Geometry: final body of the model. Coordinates: model frame, mm. A direction names the side the tool comes from. Coordinates: 2 decimals unless noted, no trailing zeros. Write each loop counter-clockwise with the first axis right and the second up, starting at its lowest first coordinate (ties: lowest second). Pieces come first, ordered by that corner, then holes. Notation, with made-up numbers: (36.5, -30) -> (92.5, -30) arc R13 cw to (92.5, -5) -> close; hole circle Ø11 at (38, 88). An arc over 180 degrees is marked (long way). One line per item, written item: value.
```python
from build123d import *

# Parameters (mm, degrees)
SKETCH1_W           = 50.8
SKETCH1_H           = 95.972651844
SKETCH1_R           = 3.175
SKETCH1_R_2         = 3.81
BOSS_EXTRUDE1_DEPTH = 6.35
SKETCH1_3_W         = 6.35
SKETCH1_3_H         = 95.972651844
BOSS_EXTRUDE2_DEPTH = 57.15
FILLET1_R           = 6.35
SKETCH2_R           = 6.096
SKETCH2_R_2         = 2.54
SKETCH2_R_3         = 3.048
CUT_EXTRUDE1_DEPTH  = 6.35
CUT_EXTRUDE2_REACH  = 99.995
SKETCH2_4_R         = 2.54
SKETCH3_W           = 31.75
SKETCH3_H           = 6.35
BOSS_EXTRUDE4_DEPTH = 30.48


with BuildPart() as part:
    # Sketch1 → Boss-Extrude1 (new body)
    with BuildSketch(Plane(origin=(0, 0, 0), x_dir=(1, 0, 0), z_dir=(0, 1, 0))):
        with Locations((0, -0.019674078)):
            Rectangle(SKETCH1_W, SKETCH1_H)
        with Locations(Location((-19.05, -41.656, 0), (0, 0, 270))):
            Circle(SKETCH1_R, mode=Mode.SUBTRACT)
        with Locations(Location((19.05, -41.656, 0), (0, 0, 270))):
            Circle(SKETCH1_R, mode=Mode.SUBTRACT)
        with Locations(Location((-19.05, 41.616651844, 0), (0, 0, 270))):
            Circle(SKETCH1_R, mode=Mode.SUBTRACT)
        with Locations(Location((0, 0, 0), (0, 0, 270))):
            Circle(SKETCH1_R_2, mode=Mode.SUBTRACT)
        with Locations(Location((19.05, 41.616651844, 0), (0, 0, 270))):
            Circle(SKETCH1_R, mode=Mode.SUBTRACT)
    extrude(amount=BOSS_EXTRUDE1_DEPTH)

    # Sketch1<3> → Boss-Extrude2 (add)
    with BuildSketch(Plane(origin=(0, 0, 0), x_dir=(1, 0, 0), z_dir=(0, 1, 0))):
        with Locations((-28.575, -0.019674078)):
            Rectangle(SKETCH1_3_W, SKETCH1_3_H)
        with Locations((28.575, -0.019674078)):
            Rectangle(SKETCH1_3_W, SKETCH1_3_H)
    extrude(amount=BOSS_EXTRUDE2_DEPTH)

    # Fillet1
    # the kernel refuses this fillet: 6.35 mm, written as the material it adds along each edge
    with BuildSketch(Plane(origin=(25.4, 6.35, 48.006), x_dir=(0, 1, 0), z_dir=(0, 0, -1))) as fillet1_piece_1_section:
        with BuildLine():
            CenterArc((FILLET1_R, -FILLET1_R), FILLET1_R, 90, 90)
            Line((0, -FILLET1_R), (0, 0))
            Line((0, 0), (FILLET1_R, 0))
        make_face()
    fillet1_piece_1 = extrude(amount=95.972651844, mode=Mode.PRIVATE)
    fillet1_piece_1 = fillet1_piece_1 - Plane(origin=(19.05, 7.801972373, 41.656), x_dir=(0, 0, 1), z_dir=(0, -1, 0)) * Cylinder(3.175, 218, mode=Mode.PRIVATE)
    fillet1_piece_1 = fillet1_piece_1 - Plane(origin=(19.05, 7.801972373, -41.616651844), x_dir=(0, 0, 1), z_dir=(0, -1, 0)) * Cylinder(3.175, 218, mode=Mode.PRIVATE)
    add(fillet1_piece_1)
    with BuildSketch(Plane(origin=(-25.4, 6.35, -47.966651844), x_dir=(1, 0, 0), z_dir=(0, 0, 1))) as fillet1_piece_2_section:
        with BuildLine():
            CenterArc((FILLET1_R, FILLET1_R), FILLET1_R, 180, 90)
            Line((0, FILLET1_R), (0, 0))
            Line((0, 0), (FILLET1_R, 0))
        make_face()
    fillet1_piece_2 = extrude(amount=95.972651844, mode=Mode.PRIVATE)
    fillet1_piece_2 = fillet1_piece_2 - Plane(origin=(-19.05, 7.801971704, 41.656), x_dir=(0, 0, 1), z_dir=(0, -1, 0)) * Cylinder(3.175, 218, mode=Mode.PRIVATE)
    fillet1_piece_2 = fillet1_piece_2 - Plane(origin=(-19.05, 7.801971704, -41.616651844), x_dir=(0, 0, 1), z_dir=(0, -1, 0)) * Cylinder(3.175, 218, mode=Mode.PRIVATE)
    add(fillet1_piece_2)
    # the kernel refuses this fillet: 6.35 mm, written as the material it takes off along each edge
    with BuildSketch(Plane(origin=(-31.75, 0, -63.841651844), x_dir=(1, 0, 0), z_dir=(0, 0, 1)), Plane(origin=(31.75, 0, 63.881), x_dir=(-1, 0, 0), z_dir=(0, 0, -1))) as fillet1_2_piece_1:
        with BuildLine():
            CenterArc((FILLET1_R, FILLET1_R), FILLET1_R, 180, 90)
            Line((0, FILLET1_R), (0, 0))
            Line((0, 0), (FILLET1_R, 0))
        make_face()
    extrude(amount=127.722651844, mode=Mode.SUBTRACT)

    # Sketch2 → Cut-Extrude1 (cut)
    # profile 1 of 6: a face of its own
    with BuildSketch(Plane(origin=(31.75, 0, 0), x_dir=(0, 0, -1), z_dir=(1, 0, 0))):
        with Locations((-22.606, 31.75)):
            Circle(SKETCH2_R)
        with Locations((-22.606, 31.75)):
            Circle(SKETCH2_R_2, mode=Mode.SUBTRACT)
    # profile 2 of 6: a face of its own
    with BuildSketch(Plane(origin=(31.75, 0, 0), x_dir=(0, 0, -1), z_dir=(1, 0, 0))):
        with Locations((-22.606, 31.75)):
            Circle(SKETCH2_R_2)
    # profile 3 of 6: a face of its own
    with BuildSketch(Plane(origin=(31.75, 0, 0), x_dir=(0, 0, -1), z_dir=(1, 0, 0))):
        with Locations((-22.606, 31.75)):
            Circle(SKETCH2_R)
    # profile 4 of 6: a face of its own
    with BuildSketch(Plane(origin=(31.75, 0, 0), x_dir=(0, 0, -1), z_dir=(1, 0, 0))):
        with Locations((-16.256, 31.75)):
            Circle(SKETCH2_R_3)
    # profile 5 of 6: a face of its own
    with BuildSketch(Plane(origin=(31.75, 0, 0), x_dir=(0, 0, -1), z_dir=(1, 0, 0))):
        with Locations((-22.606, 31.75)):
            Circle(SKETCH2_R)
    # profile 6 of 6: a face of its own
    with BuildSketch(Plane(origin=(31.75, 0, 0), x_dir=(0, 0, -1), z_dir=(1, 0, 0))):
        with Locations((-16.256, 31.75)):
            Circle(SKETCH2_R_3)
    extrude(amount=-CUT_EXTRUDE1_DEPTH, mode=Mode.SUBTRACT)

    # Cut-Extrude2: up to this face of the body (flat: up to its plane)
    cut_extrude2_end = Plane(part.part.faces().sort_by_distance((-31.75, 31.75, 0.019674078))[0])
    # Sketch2<4> → Cut-Extrude2 (cut, up to the picked face)
    with BuildSketch(Plane(origin=(31.75, 0, 0), x_dir=(0, 0, -1), z_dir=(1, 0, 0)), mode=Mode.PRIVATE) as cut_extrude2_sk1:
        with Locations((22.606, 31.75)):
            Circle(SKETCH2_4_R)
    cut_extrude2_tool1 = split(extrude(cut_extrude2_sk1.sketch, amount=-CUT_EXTRUDE2_REACH, mode=Mode.PRIVATE), bisect_by=cut_extrude2_end, keep=Keep.BOTH, mode=Mode.PRIVATE)
    # Sketch2<4> → Cut-Extrude2 (cut, up to the picked face)
    with BuildSketch(Plane(origin=(31.75, 0, 0), x_dir=(0, 0, -1), z_dir=(1, 0, 0)), mode=Mode.PRIVATE) as cut_extrude2_sk2:
        with Locations((-22.606, 31.75)):
            Circle(SKETCH2_4_R)
    cut_extrude2_tool2 = split(extrude(cut_extrude2_sk2.sketch, amount=-CUT_EXTRUDE2_REACH, mode=Mode.PRIVATE), bisect_by=cut_extrude2_end, keep=Keep.BOTH, mode=Mode.PRIVATE)
    add(cut_extrude2_tool1.solids().sort_by(Axis((31.75, 31.75, -22.606), (-1, 0, 0)))[0], mode=Mode.SUBTRACT)
    add(cut_extrude2_tool2.solids().sort_by(Axis((31.75, 31.75, 22.606), (-1, 0, 0)))[0], mode=Mode.SUBTRACT)

    # Sketch3 → Boss-Extrude4 (add)
    with BuildSketch(Plane.ZY.offset(-25.4)):
        with Locations((18.766859732, 22.479)):
            Rectangle(SKETCH3_W, SKETCH3_H)
        with Locations((18.766859732, 41.021)):
            Rectangle(SKETCH3_W, SKETCH3_H)
    extrude(amount=BOSS_EXTRUDE4_DEPTH)


solid = part.part
```
(1) Reachability of faces 1 (the flat face through (-25.4, 35, 1)), 2 (the flat face through (10, 19.304, 19)), 3 (the flat face through (10, 41, 2.892)), 4 (the flat face through (10, 22, 34.642)) from +Z, -Z, +X, -X, +Y, -Y: full face, straight path, thin tool, end or side. Return the list, or none.
Responses:
face 1: +Z, -Z, +Y
face 2: +Z, -Z
face 3: -Z, +Y
face 4: +Z, +Y
(2) Section B-B (y = 31.75). Return the cut outline in (x, z), then the cut area to 3 significant figures.
Responses:
outline: (-31.75, -47.97) -> (-25.4, -47.97) -> (-25.4, -25.15) -> (-31.75, -25.15) -> close; (-31.75, -20.07) -> (-25.4, -20.07) -> (-25.4, 20.07) -> (-31.75, 20.07) -> close; (-31.75, 25.15) -> (-25.4, 25.15) -> (-25.4, 48.01) -> (-31.75, 48.01) -> close; (25.4, -47.97) -> (31.75, -47.97) -> (31.75, -25.15) -> (25.4, -25.15) -> close; (25.4, -20.07) -> (31.75, -20.07) -> (31.75, 13.21) -> (25.4, 13.21) -> close; (25.4, 28.7) -> (31.75, 28.7) -> (31.75, 48.01) -> (25.4, 48.01) -> close
area: 1,020 mm2
(3) Section A-A (z = 0). Return the cut outline in (x, y), then the cut area to 4 significant figures.
Responses:
outline: (-31.75, 6.35) arc R6.35 ccw to (-25.4, 0) -> (-3.81, 0) -> (-3.81, 6.35) -> (-19.05, 6.35) arc R6.35 cw to (-25.4, 12.7) -> (-25.4, 57.15) -> (-31.75, 57.15) -> close; (3.81, 0) -> (25.4, 0) arc R6.35 ccw to (31.75, 6.35) -> (31.75, 57.15) -> (25.4, 57.15) -> (25.4, 12.7) arc R6.35 cw to (19.05, 6.35) -> (3.81, 6.35) -> close
area: 1,000 mm2
(4) Section C-C (x = 6.5). Return the cut outline in (y, z), then the cut area to 3 significant figures.
Responses:
outline: (0, -47.97) -> (6.35, -47.97) -> (6.35, 48.01) -> (0, 48.01) -> close; (19.3, 2.89) -> (25.65, 2.89) -> (25.65, 34.64) -> (19.3, 34.64) -> close; (37.85, 2.89) -> (44.2, 2.89) -> (44.2, 34.64) -> (37.85, 34.64) -> close
area: 1,010 mm2
(5) Pull-direction query (Y, two-part tool) for faces 5 (the flat face through (10, 44.196, 19)), 6 (the flat face through (10, 37.846, 19)), 7 (the flat face through (5, 0, -1)); classes: released by +Y, released by -Y, zero draft, split by the parting line, or undercut.
Responses:
face 5: released by +Y
face 6: undercut
face 7: released by -Y
(6) First-contact query: pin 1 (12 mm diameter, centred on x = -11.5, z = -8, fed in from +Y); pin 2 (5 mm diameter, centred on x = 11, y = 22, fed in from -Z); pin 3 (9 mm diameter, centred on x = 10.5, z = 11.5, fed in from +Y). Flat tips, straight axial feed; report the tip coordinate or a pass-through.
Responses:
pin 1: stops at y = 6.35
pin 2: stops at z = 2.89
pin 3: stops at y = 44.2
(7) Section D-D (y = 11). Return the cut outline in (x, z), then the cut area to 3 significant figures.
Responses:
outline: (-31.75, -47.97) -> (-25.17, -47.97) -> (-25.17, 48.01) -> (-31.75, 48.01) -> close; (25.17, -47.97) -> (31.75, -47.97) -> (31.75, 48.01) -> (25.17, 48.01) -> close
area: 1,260 mm2
(8) Line query: line 1 (Y direction, x = 1.5, z = 27); line 2 (Z direction, x = -19, y = 2); line 3 (X direction, y = 29, z = 40). Output: solid intervals per line, ascending. Write a range as [from, to].
Responses:
line 1: y = [0, 6.35], [19.3, 25.65], [37.85, 44.2]
line 2: z = [-47.97, -44.79], [-38.44, 38.48], [44.83, 48.01]
line 3: x = [-31.75, -25.4], [25.4, 31.75]
